from build123d import *

# Parameters (mm, degrees)
SKETCH2_W           = 66
SKETCH2_H           = 25
BOSS_EXTRUDE1_DEPTH = 12
SKETCH3_W           = 64.4
SKETCH3_H           = 23.4
CUT_EXTRUDE1_DEPTH  = 11.2
SKETCH5_R           = 5
CUT_EXTRUDE2_DEPTH  = 69.23672032


with BuildPart() as part:
    # Sketch2 → Boss-Extrude1 (new body)
    with BuildSketch(Plane.XY):
        Rectangle(SKETCH2_W, SKETCH2_H)
    extrude(amount=BOSS_EXTRUDE1_DEPTH)

    # Sketch3 → Cut-Extrude1 (cut)
    with BuildSketch(Plane.XY.offset(12)):
        Rectangle(SKETCH3_W, SKETCH3_H)
    extrude(amount=-CUT_EXTRUDE1_DEPTH, mode=Mode.SUBTRACT)

    # Sketch5 → Cut-Extrude2 (cut, through all)
    with BuildSketch(Plane(origin=(33, 0, 0), x_dir=(0, 0, -1), z_dir=(1, 0, 0))):
        with Locations((-12, 0)):
            Circle(SKETCH5_R)
    extrude(amount=-CUT_EXTRUDE2_DEPTH, mode=Mode.SUBTRACT)


solid = part.part
Can you work these out from the model? Positions are in its coordinate system, mm. A direction names the side the tool comes from. Give positions to 0.01 mm unless a question says otherwise; leave off trailing zeros. Order: outer loops, then holes, each group sorted by start corner. A loop starts at its lowest first (then second) coordinate and runs counter-clockwise, first axis right, second up. Notation, with made-up numbers: M 35.25,9.5 L 85.25,9.5 A8 ccw 85.25,15.5 Z; hole C -9,66 d9. An arc over 180 degrees is marked long. Use a Markdown table: item, result. Add a question column.
Item 1: Suppose I cut it at B-B (y = 3). List the corners of the cut face in (x, z) for me.
Item 2: We'd pull the mould along X, two halves only. Please class faces 1 (the flat face through (0, 11.7, 6)), 2 (the flat face through (0, -12.5, 6)), 3 (the flat face through (-33, 0, 6)), 4 (the flat face through (0, 0, 0.8)): +X half, -X half, draft (parallel to the pull), parting line (faces both ways), or undercut.
Item 3: If I drill on L1, parallel to X at y = 7.75, z = 10; L2, parallel to Y at x = -27, z = 6.25; L3, parallel to Z at x = -21, y = 11.5, over which ranges is the centre line in solid material (lowest first)? Write a range as [from, to].
Item 4: For faces 5 (the flat face through (0, 12, 12)), 6 (the flat face through (-32.2, 0, 6)), which set-ups out of +Z, -Z, +X, -X, +Y, -Y let a thin tool reach every point of the face, with its end or its side?
Item 5: Suppose I cut it at D-D (z = 8.5). List the corners of the cut face in (x, y) for me.
Item 6: Suppose I cut it at A-A (z = 3). List the corners of the cut face in (x, y) for me.
Item 7: Will these pins go through, and if not, where does the flat tip stop? pin 1 (12 mm diameter, centred on x = -24, y = -2, fed in from +Z); pin 2 (1.5 mm diameter, centred on y = 2, z = 9, fed in from -X).
Item 8: Suppose I cut it at C-C (x = 6). List the corners of the cut face in (y, z) for me.
Answer sheet:
| question | item | result |
|---|---|---|
| 1 | outline | M -33,0 L 33,0 L 33,8 L 32.2,8 L 32.2,0.8 L -32.2,0.8 L -32.2,8 L -33,8 Z |
| 2 | face 1 | undercut |
| 2 | face 2 | draft |
| 2 | face 3 | -X half |
| 2 | face 4 | undercut |
| 3 | L1 | x = [-33, -32.2], [32.2, 33] |
| 3 | L2 | y = [-12.5, -11.7], [11.7, 12.5] |
| 3 | L3 | z = [0, 0.8] |
| 4 | face 5 | +Z, +X, -X, +Y, -Y |
| 4 | face 6 | +Z |
| 5 | outline | M -33,-12.5 L 33,-12.5 L 33,-3.57 L 32.2,-3.57 L 32.2,-11.7 L -32.2,-11.7 L -32.2,-3.57 L -33,-3.57 Z; M -33,3.57 L -32.2,3.57 L -32.2,11.7 L 32.2,11.7 L 32.2,3.57 L 33,3.57 L 33,12.5 L -33,12.5 Z |
| 6 | outline | M -33,-12.5 L 33,-12.5 L 33,12.5 L -33,12.5 Z; hole M -32.2,-11.7 L 32.2,-11.7 L 32.2,11.7 L -32.2,11.7 Z |
| 7 | pin 1 | stops at z = 0.8 |
| 7 | pin 2 | passes through |
| 8 | outline | M -12.5,0 L 12.5,0 L 12.5,12 L 11.7,12 L 11.7,0.8 L -11.7,0.8 L -11.7,12 L -12.5,12 Z |
